Read the model definition and answer for the solid it produces. Units are mm, in the model's axes. A direction names the side the tool comes from. Coordinates: 2 decimals unless noted, no trailing zeros. Order: outer loops, then holes, each group sorted by start corner. A loop starts at its lowest first (then second) coordinate and runs counter-clockwise, first axis right, second up. Notation, with made-up numbers: M 18.25,1.5 L 40.25,1.5 A19 ccw 40.25,10.5 Z; hole C -38,-17 d1. An arc over 180 degrees is marked long. Use a Markdown table: item, result. Add a question column.
1) Find section D-D on z = -50.5. Write down the section's boundary in (x, y), plus the area to 3 significant figures.
2) The mould has two halves that part along X. Classify faces 4 (the face through (138, 98, 0)), 5 (the face through (0, 68, -39)), 6 (the face through (138, 98, 15)): released by +X, released by -X, zero draft, split by the parting line, or undercut.
3) Find section C-C on y = 70.5. Write down the section's boundary in (x, z), plus the area to 3 significant figures.
4) Find section B-B on x = 213.5. Write down the section's boundary in (y, z), plus the area to 3 significant figures.
5) For faces 1 (the face through (15, 68, -39)), 2 (the face through (210, 68, -87)), 3 (the face through (35, 67, -95)), determine the directions among +Z, -Z, +X, -X, +Y, -Y from which every point of the face is accessible in a straight line to the end or side of a thin tool.
6) Each of these flat-tipped pins is pushed along its axis until it touches: pin 1 Ø7.5 at (y, z) = (52, -90.5) entering from -X; pin 2 Ø10 at (x, z) = (209.5, -83.5) entering from -Y. Where does it stop, or does it pass through?
7) Find the intervals of material crossed by probe 1 along Z at (x, y) = (243, 63); probe 2 along X at (y, z) = (102, -4); probe 3 along Z at (x, y) = (113.5, 95), in increasing order. Write a range as [from, to].
8) Find section A-A on z = -88. Write down the section's boundary in (x, y), plus the area to 3 significant figures.
from build123d import *

# Parameters (mm, degrees)
F0_W      = 280
F0_H      = 135
F1_DEPTH  = 15
F3_DEPTH  = 15
F4_W      = 135
F4_H      = 15
F5_DEPTH  = 15
F7_DEPTH  = 110.001
F9_DEPTH  = 55
F11_DEPTH = 55
F13_DEPTH = 25


with BuildPart() as f1:
    # F0 (on Top) → F1 (new body)
    with BuildSketch(Plane.XY):
        with Locations((140, 67.5)):
            Rectangle(F0_W, F0_H)
    extrude(amount=F1_DEPTH)

    # F2 (on face) → F3 (join)
    with BuildSketch(Plane(origin=(0, 0, 0), x_dir=(0, -1, 0), z_dir=(-1, 0, 0))):
        Polygon((0, 0), (-135, 0), (-107.5, -95), (-67.5, -95), (-27.5, -95), align=None)
    extrude(amount=-F3_DEPTH)

    # F4 (on face) → F5 (join)
    with BuildSketch(Plane.YZ.offset(280)):
        Polygon((27.5, -95), (67.5, -95), (107.5, -95), (135, 0), (0, 0), align=None)
        with Locations((67.5, 7.5)):
            Rectangle(F4_W, F4_H)
    extrude(amount=-F5_DEPTH)

    # F6 (on face) → F7 (cut, through all)
    with BuildSketch(Plane.XY.offset(15)):
        with BuildLine():
            ThreePointArc((112.9769395589, 54.4710244302), (140, 37.5), (167.0230604411, 54.4710244302))
            Line((167.0230604411, 54.4710244302), (140, 67.5))
            Line((140, 67.5), (112.9769395589, 54.4710244302))
        make_face()
        with BuildLine():
            Line((140, 67.5), (167.0230604411, 54.4710244302))
            ThreePointArc((167.0230604411, 54.4710244302), (169.2462973146, 60.8176281618), (170, 67.5))
            ThreePointArc((170, 67.5), (169.2462973146, 74.1823718382), (167.0230604411, 80.5289755698))
            Line((167.0230604411, 80.5289755698), (140, 67.5))
        make_face()
        with BuildLine():
            Line((112.9769395589, 54.4710244302), (140, 67.5))
            Line((140, 67.5), (112.9769395589, 80.5289755698))
            ThreePointArc((112.9769395589, 80.5289755698), (110, 67.5), (112.9769395589, 54.4710244302))
        make_face()
        with BuildLine():
            Line((112.9769395589, 80.5289755698), (140, 67.5))
            Line((140, 67.5), (167.0230604411, 80.5289755698))
            ThreePointArc((167.0230604411, 80.5289755698), (140, 97.5), (112.9769395589, 80.5289755698))
        make_face()
    extrude(amount=-F7_DEPTH, mode=Mode.SUBTRACT)

    # F8 (on face) → F9 (join)
    with BuildSketch(Plane.YZ.offset(15)):
        Polygon((111.8421052632, -80), (27.5, -80), (23.1578947368, -80), (27.5, -95), (107.5, -95), align=None)
    extrude(amount=F9_DEPTH)

    # F10 (on face) → F11 (join)
    with BuildSketch(Plane(origin=(265, 0, 0), x_dir=(0, -1, 0), z_dir=(-1, 0, 0))):
        Polygon((-107.5, -95), (-67.5, -95), (-67.5, -80), (-111.8421052632, -80), align=None)
        Polygon((-67.5, -80), (-67.5, -95), (-27.5, -95), (-23.1578947368, -80), align=None)
    extrude(amount=F11_DEPTH)

    # F12 (on face) → F13 (cut)
    with BuildSketch(Plane(origin=(0, 0, -95), x_dir=(1, 0, 0), z_dir=(0, 0, -1))):
        with BuildLine():
            ThreePointArc((35, -97.5), (42.0710678119, -94.5710678119), (45, -87.5))
            Line((45, -87.5), (35, -87.5))
            Line((35, -87.5), (35, -97.5))
        make_face()
        with BuildLine():
            Line((245, -77.5), (245, -87.5))
            Line((245, -87.5), (255, -87.5))
            ThreePointArc((255, -87.5), (252.0710678119, -80.4289321881), (245, -77.5))
        make_face()
        with BuildLine():
            ThreePointArc((245, -77.5), (237.9289321881, -80.4289321881), (235, -87.5))
            Line((235, -87.5), (245, -87.5))
            Line((245, -87.5), (245, -77.5))
        make_face()
        with BuildLine():
            Line((255, -87.5), (245, -87.5))
            Line((245, -87.5), (245, -97.5))
            ThreePointArc((245, -97.5), (252.0710678119, -94.5710678119), (255, -87.5))
        make_face()
        with BuildLine():
            Line((245, -87.5), (235, -87.5))
            ThreePointArc((235, -87.5), (237.9289321881, -94.5710678119), (245, -97.5))
            Line((245, -97.5), (245, -87.5))
        make_face()
        with BuildLine():
            Line((35, -87.5), (45, -87.5))
            ThreePointArc((45, -87.5), (42.0710678119, -80.4289321881), (35, -77.5))
            Line((35, -77.5), (35, -87.5))
        make_face()
        with BuildLine():
            Line((35, -97.5), (35, -87.5))
            Line((35, -87.5), (25, -87.5))
            ThreePointArc((25, -87.5), (27.9289321881, -94.5710678119), (35, -97.5))
        make_face()
        with BuildLine():
            Line((35, -87.5), (35, -77.5))
            ThreePointArc((35, -77.5), (27.9289321881, -80.4289321881), (25, -87.5))
            Line((25, -87.5), (35, -87.5))
        make_face()
        with BuildLine():
            ThreePointArc((35, -57.5), (42.0710678119, -54.5710678119), (45, -47.5))
            Line((45, -47.5), (35, -47.5))
            Line((35, -47.5), (35, -57.5))
        make_face()
        with BuildLine():
            Line((35, -57.5), (35, -47.5))
            Line((35, -47.5), (25, -47.5))
            ThreePointArc((25, -47.5), (27.9289321881, -54.5710678119), (35, -57.5))
        make_face()
        with BuildLine():
            Line((35, -47.5), (35, -37.5))
            ThreePointArc((35, -37.5), (27.9289321881, -40.4289321881), (25, -47.5))
            Line((25, -47.5), (35, -47.5))
        make_face()
        with BuildLine():
            ThreePointArc((45, -47.5), (42.0710678119, -40.4289321881), (35, -37.5))
            Line((35, -37.5), (35, -47.5))
            Line((35, -47.5), (45, -47.5))
        make_face()
        with BuildLine():
            Line((245, -47.5), (235, -47.5))
            ThreePointArc((235, -47.5), (237.9289321881, -54.5710678119), (245, -57.5))
            Line((245, -57.5), (245, -47.5))
        make_face()
        with BuildLine():
            Line((255, -47.5), (245, -47.5))
            Line((245, -47.5), (245, -57.5))
            ThreePointArc((245, -57.5), (252.0710678119, -54.5710678119), (255, -47.5))
        make_face()
        with BuildLine():
            ThreePointArc((255, -47.5), (252.0710678119, -40.4289321881), (245, -37.5))
            Line((245, -37.5), (245, -47.5))
            Line((245, -47.5), (255, -47.5))
        make_face()
        with BuildLine():
            Line((245, -47.5), (245, -37.5))
            ThreePointArc((245, -37.5), (237.9289321881, -40.4289321881), (235, -47.5))
            Line((235, -47.5), (245, -47.5))
        make_face()
    extrude(amount=-F13_DEPTH, mode=Mode.SUBTRACT)


solid = f1.part
Check result:
| question | item | result |
|---|---|---|
| 1 | outline | M 0,14.62 L 15,14.62 L 15,120.38 L 0,120.38 Z; M 265,14.62 L 280,14.62 L 280,120.38 L 265,120.38 Z |
| 1 | area | 3,170 mm2 |
| 2 | face 4 | undercut |
| 2 | face 5 | released by -X |
| 2 | face 6 | zero draft |
| 3 | outline | M 0,-95 L 70,-95 L 70,-80 L 15,-80 L 15,0 L 110.15,0 L 110.15,15 L 0,15 Z; M 169.85,0 L 265,0 L 265,-80 L 210,-80 L 210,-95 L 280,-95 L 280,15 L 169.85,15 Z |
| 3 | area | 7,800 mm2 |
| 4 | outline | M 0,0 L 135,0 L 135,15 L 0,15 Z; M 23.16,-80 L 27.5,-95 L 107.5,-95 L 111.84,-80 Z |
| 4 | area | 3,290 mm2 |
| 5 | face 1 | +Y, -Y |
| 5 | face 2 | -Z, +Y, -Y |
| 5 | face 3 | -Z, +X, -X, +Y, -Y |
| 6 | pin 1 | stops at x = 0 |
| 6 | pin 2 | stops at y = 23.16 |
| 7 | probe 1 | z = [-95, -80], [0, 15] |
| 7 | probe 2 | x = [0, 15], [265, 280] |
| 7 | probe 3 | z = [0, 15] |
| 8 | outline | M 0,25.47 L 70,25.47 L 70,109.53 L 0,109.53 Z; M 210,25.47 L 280,25.47 L 280,109.53 L 210,109.53 Z; hole C 35,47.5 d20; hole C 35,87.5 d20; hole C 245,47.5 d20; hole C 245,87.5 d20 |
| 8 | area | 10,500 mm2 |
